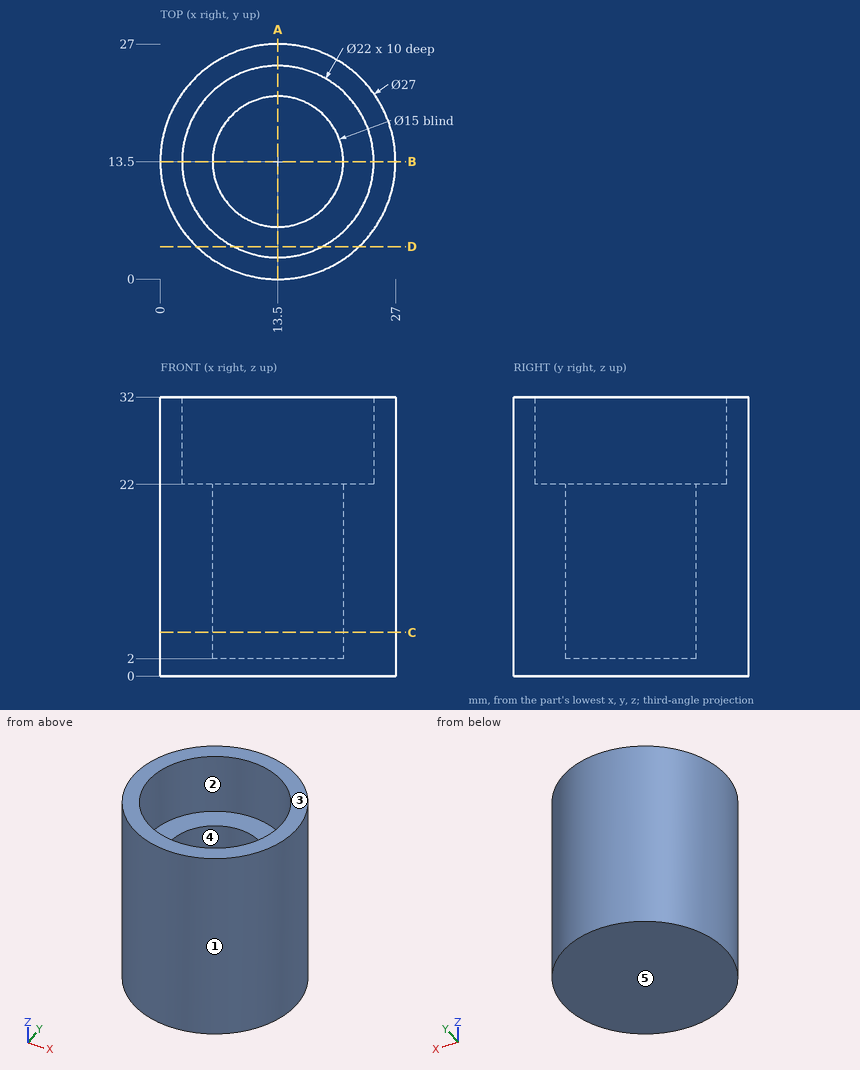
Here's the drawing with two shaded views (mm, measured from the low corner). I have some questions. A direction names the side the tool comes from. Coordinates: 2 decimals unless noted, no trailing zeros. Loops run counter-clockwise (first coordinate to the right, second up) from the corner with the lowest first, then second, coordinate; pieces in that order, holes last. Notation, with made-up numbers: M -16.75,-32.75 L 18.25,-32.75 A13 ccw 18.25,-27.75 Z; hole C 66,-39 d7. An arc over 180 degrees is marked long. Answer as CSV lines item,"result". Start each with the question number.
1. If I drill on probe 1 along Y at (x, z) = (13.5, 27); probe 2 along Y at (x, z) = (13.5, 2.5); probe 3 along Z at (x, y) = (5.5, 14), over which ranges is the centre line in solid material (lowest first)? Write a range as [from, to].
2. For the marked faces 4 and 5, which set-ups out of +Z, -Z, +X, -X, +Y, -Y let a thin tool reach every point of the face, with its end or its side?
3. Thinking about a two-plate mould opening in X: for the marked faces 1, 2 and 3, which applies, +X half, -X half, draft (parallel to the pull), parting line (faces both ways), or undercut?
4. Suppose I cut it at D-D, the plane y = 3.75. List the corners of the cut face in (x, z) for me, plus the area to 3 significant figures.
5. Suppose I cut it at A-A, the plane x = 13.5. List the corners of the cut face in (y, z) for me, plus the area to 3 significant figures.
6. For pin 1 Ø6 at (x, y) = (9, 15.5) entering from +Z; pin 2 Ø10 at (x, z) = (6.5, 24.5) entering from -Y; pin 3 Ø1 at (x, z) = (15.5, 19.5) entering from -Y, each with a flat end and sliding along its axis, tell me the tip position at first contact or that it passes through.
7. Suppose I cut it at C-C, the plane z = 5. List the corners of the cut face in (x, y) for me.
Output:
1,probe 1,"y = [0, 2.5], [24.5, 27]"
1,probe 2,"y = [0, 6], [21, 27]"
1,probe 3,"z = [0, 22]"
2,face 4,"+Z"
2,face 5,"-Z, +X, -X, +Y, -Y"
3,face 1,"parting line"
3,face 2,"undercut"
3,face 3,"draft"
4,outline,"M 4.16,0 L 22.84,0 L 22.84,32 L 18.59,32 L 18.59,22 L 8.41,22 L 8.41,32 L 4.16,32 Z"
4,area,"496 mm^2"
5,outline,"M 0,0 L 27,0 L 27,32 L 24.5,32 L 24.5,22 L 21,22 L 21,2 L 6,2 L 6,22 L 2.5,22 L 2.5,32 L 0,32 Z"
5,area,"344 mm^2"
6,pin 1,"stops at z = 22"
6,pin 2,"stops at y = 0.15"
6,pin 3,"stops at y = 0.08"
7,outline,"C 13.5,13.5 d27; hole C 13.5,13.5 d15"
